```python
from build123d import *

# Parameters (mm, degrees)
CROQUIS1_W                   = 7.5
CROQUIS1_H                   = 5.9
CROQUIS1_W_2                 = 0.64
CROQUIS1_H_2                 = 0.8
SALIENTE_EXTRUIR1_DEPTH      = 1
CROQUIS2_W                   = 7.5
CROQUIS2_H                   = 5.9
CROQUIS2_W_2                 = 6
CROQUIS2_H_2                 = 4.4
SALIENTE_EXTRUIR2_DEPTH      = 6
CORTAR_EXTRUIR1_DEPTH        = 9
CORTAR_EXTRUIR2_DEPTH        = 2
SALIENTE_EXTRUIR3_DEPTH      = 6.5
SALIENTE_EXTRUIR3_DEPTH_BACK = 3.4
CROQUIS5_W                   = 0.64
CROQUIS5_H                   = 0.8


with BuildPart() as part:
    # Croquis1 → Saliente-Extruir1 (new body)
    with BuildSketch(Plane(origin=(0, 0, 0), x_dir=(1, 0, 0), z_dir=(0, 1, 0))):
        with Locations((1.27, 0.42)):
            Rectangle(CROQUIS1_W, CROQUIS1_H)
        Rectangle(CROQUIS1_W_2, CROQUIS1_H_2, mode=Mode.SUBTRACT)
        with Locations((2.54, 0)):
            Rectangle(CROQUIS1_W_2, CROQUIS1_H_2, mode=Mode.SUBTRACT)
    extrude(amount=SALIENTE_EXTRUIR1_DEPTH)

    # Croquis2 → Saliente-Extruir2 (add)
    with BuildSketch(Plane(origin=(0, 1, 0), x_dir=(1, 0, 0), z_dir=(0, 1, 0))):
        with Locations((1.27, 0.42)):
            Rectangle(CROQUIS2_W, CROQUIS2_H)
        with Locations((1.27, 0.42)):
            Rectangle(CROQUIS2_W_2, CROQUIS2_H_2, mode=Mode.SUBTRACT)
    extrude(amount=SALIENTE_EXTRUIR2_DEPTH)

    # Croquis3 → Cortar-Extruir1 (cut)
    with BuildSketch(Plane.ZY.offset(2.48)):
        with BuildLine():
            Line((1.78, 7), (1.78, 4.35))
            ThreePointArc((1.78, 4.35), (1.604264069, 3.925735931), (1.18, 3.75))
            Line((1.18, 3.75), (0.78, 3.75))
            Line((0.78, 3.75), (0.78, 7))
            Line((0.78, 7), (1.78, 7))
        make_face()
    extrude(amount=-CORTAR_EXTRUIR1_DEPTH, mode=Mode.SUBTRACT)

    # Croquis4 → Cortar-Extruir2 (cut)
    with BuildSketch(Plane.XY.offset(2.53)):
        with BuildLine():
            Line((-0.48, 3.85), (-0.48, 7))
            Line((-0.48, 7), (3.02, 7))
            Line((3.02, 7), (3.02, 3.85))
            ThreePointArc((3.02, 3.85), (2.844264069, 3.425735931), (2.42, 3.25))
            Line((2.42, 3.25), (1.266494324, 3.25))
            Line((1.266494324, 3.25), (0.12, 3.25))
            ThreePointArc((0.12, 3.25), (-0.304264069, 3.425735931), (-0.48, 3.85))
        make_face()
    extrude(amount=-CORTAR_EXTRUIR2_DEPTH, mode=Mode.SUBTRACT)

    # Croquis5 → Saliente-Extruir3 (add, two sides: drawn at the far end of the back side and taken through both)
    with BuildSketch(Plane(origin=(0, 0, 0), x_dir=(1, 0, 0), z_dir=(0, 1, 0)).offset(-SALIENTE_EXTRUIR3_DEPTH_BACK)):
        with Locations((2.54, 0)):
            Rectangle(CROQUIS5_W, CROQUIS5_H)
        Rectangle(CROQUIS5_W, CROQUIS5_H)
    extrude(amount=SALIENTE_EXTRUIR3_DEPTH + SALIENTE_EXTRUIR3_DEPTH_BACK)


solid = part.part
```
Input: part model. Units: mm. Frame: model coordinates. A direction names the side the tool comes from. Coordinates: 2 decimals unless noted, no trailing zeros. Order: outer loops, then holes, each group sorted by start corner. A loop starts at its lowest first (then second) coordinate and runs counter-clockwise, first axis right, second up. Notation, with made-up numbers: (88, 89) - (123, 89) arc R14 ccw to (123, 104) - close; hole circle Ø3 at (79, 29). An arc over 180 degrees is marked (long way). Return JSON: item names as keys, results as strings.
Q1. Ray query, probe 1 along X at (y, z) = (6.5, -2.55); probe 2 along X at (y, z) = (4.75, 2); probe 3 along Z at (x, y) = (4, 6.5). Return the intervals inside material, ascending.
The answers:
{"probe 1": "x = -2.48 to -1.73, 4.27 to 5.02", "probe 2": "x = -2.48 to -0.48, 3.02 to 5.02", "probe 3": "z = -3.37 to -2.62, 1.78 to 2.53"}
Q2. Access query for faces 1 (the flat face through (1, 7, -3)), 2 (the flat face through (-1.73, 4, 0)). Directions: +Z, -Z, +X, -X, +Y, -Y. A direction counts if a zero-diameter tool reaches every point of the face in a straight line with its end or side. Return the directions, or none.
The answers:
{"face 1": "+Z, -Z, +X, -X, +Y", "face 2": "+Y"}
Q3. Cut plane B-B (y = -0.5). Return loops of the section in (x, z), then the cut area to 3 significant figures.
The answers:
{"outline": "(-0.32, -0.4) - (0.32, -0.4) - (0.32, 0.4) - (-0.32, 0.4) - close; (2.22, -0.4) - (2.86, -0.4) - (2.86, 0.4) - (2.22, 0.4) - close", "area": "1.02 mm2"}
Q4. Draft query along Z for faces 3 (the flat face through (1, 3, 2.53)), 4 (the flat face through (1, 3, 1.78)), 5 (the flat face through (-2.48, 3, 0)). Return one class per face: +Z half, -Z half, draft (parallel to the pull), parting line (faces both ways), or undercut.
The answers:
{"face 3": "+Z half", "face 4": "undercut", "face 5": "draft"}
Q5. Cut plane D-D (y = 6). Return loops of the section in (x, z).
The answers:
{"outline": "(-2.48, -3.37) - (5.02, -3.37) - (5.02, 0.78) - (4.27, 0.78) - (4.27, -2.62) - (-1.73, -2.62) - (-1.73, 0.78) - (-2.48, 0.78) - close; (-2.48, 1.78) - (-0.48, 1.78) - (-0.48, 2.53) - (-2.48, 2.53) - close; (-0.32, -0.4) - (0.32, -0.4) - (0.32, 0.4) - (-0.32, 0.4) - close; (2.22, -0.4) - (2.86, -0.4) - (2.86, 0.4) - (2.22, 0.4) - close; (3.02, 1.78) - (5.02, 1.78) - (5.02, 2.53) - (3.02, 2.53) - close"}
Q6. First-contact query: pin 1 (0.5 mm diameter, centred on x = 0, y = -1.5, fed in from +Z); pin 2 (0.6 mm diameter, centred on y = -2, z = 0, fed in from -X). Flat tips, straight axial feed; report the tip coordinate or a pass-through.
The answers:
{"pin 1": "stops at z = 0.4", "pin 2": "stops at x = -0.32"}
Q7. Cut plane C-C (z = -0.85). Return loops of the section in (x, y).
The answers:
{"outline": "(-2.48, 0) - (5.02, 0) - (5.02, 7) - (4.27, 7) - (4.27, 1) - (-1.73, 1) - (-1.73, 7) - (-2.48, 7) - close"}
Q8. Cut plane A-A (y = 1.75). Return loops of the section in (x, z).
The answers:
{"outline": "(-2.48, -3.37) - (5.02, -3.37) - (5.02, 2.53) - (-2.48, 2.53) - close; (-0.32, -0.4) - (0.32, -0.4) - (0.32, 0.4) - (-0.32, 0.4) - close; (2.22, -0.4) - (2.86, -0.4) - (2.86, 0.4) - (2.22, 0.4) - close; hole (-1.73, -2.62) - (4.27, -2.62) - (4.27, 1.78) - (-1.73, 1.78) - close"}
